For this review, take the finished solid that the model builds, in its own axes (mm). Face numbers are marked on the shaded views. A direction names the side the tool comes from. Round coordinates to 2 decimals unless told otherwise and drop trailing zeros. Order: outer loops, then holes, each group sorted by start corner. A loop starts at its lowest first (then second) coordinate and runs counter-clockwise, first axis right, second up. Notation, with made-up numbers: M 56,-3.5 L 115,-3.5 A21 ccw 115,0.5 Z; hole C -16,42 d5. An arc over 180 degrees is marked long. Use a Markdown table: item, result.
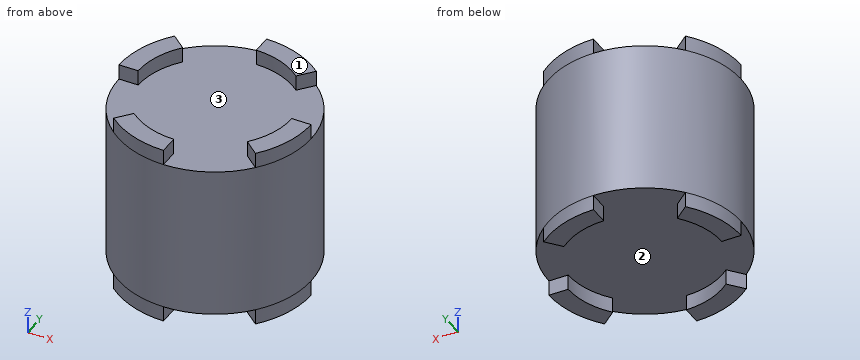
from build123d import *

# Parameters (mm, degrees)
SKETCH1_R           = 25
BOSS_EXTRUDE1_DEPTH = 20
BOSS_EXTRUDE2_START = 4
BOSS_EXTRUDE2_DEPTH = 4


with BuildPart() as part:
    # Sketch1 → Boss-Extrude1 (new, symmetric)
    with BuildSketch(Plane.XY):
        Circle(SKETCH1_R)
    extrude(amount=BOSS_EXTRUDE1_DEPTH, both=True)

    # Sketch2 → Boss-Extrude2 (add)
    with BuildSketch(Plane.XY.offset(20).offset(BOSS_EXTRUDE2_START)):
        with BuildLine():
            Line((-25, 0), (-20, 0))
            ThreePointArc((-20, 0), (-18.793852416, 6.840402867), (-15.320888862, 12.855752194))
            Line((-15.320888862, 12.855752194), (-19.151111078, 16.069690242))
            ThreePointArc((-19.151111078, 16.069690242), (-23.49231552, 8.550503583), (-25, 0))
        make_face()
        with BuildLine():
            Line((16.069690242, 19.151111078), (12.855752194, 15.320888862))
            ThreePointArc((12.855752194, 15.320888862), (6.840402867, 18.793852416), (0, 20))
            Line((0, 20), (0, 25))
            ThreePointArc((0, 25), (8.550503583, 23.49231552), (16.069690242, 19.151111078))
        make_face()
        with BuildLine():
            Line((25, 0), (20, 0))
            ThreePointArc((20, 0), (18.793852416, -6.840402867), (15.320888862, -12.855752194))
            Line((15.320888862, -12.855752194), (19.151111078, -16.069690242))
            ThreePointArc((19.151111078, -16.069690242), (23.49231552, -8.550503583), (25, 0))
        make_face()
        with BuildLine():
            Line((0, -20), (0, -25))
            ThreePointArc((0, -25), (-8.550503583, -23.49231552), (-16.069690242, -19.151111078))
            Line((-16.069690242, -19.151111078), (-12.855752194, -15.320888862))
            ThreePointArc((-12.855752194, -15.320888862), (-6.840402867, -18.793852416), (0, -20))
        make_face()
    boss_extrude2 = extrude(amount=-BOSS_EXTRUDE2_DEPTH)

    # Mirror1: Boss-Extrude2 across plane
    add(boss_extrude2.mirror(Plane.XY))


solid = part.part
Q1. Machinability: for the marked faces 1, 2 and 3, which of the approach directions +Z, -Z, +X, -X, +Y, -Y give a long, thin tool a straight path to every point of the face, cutting with its end or side? Answer none if there is none.
Determined:
| item | result |
|---|---|
| face 1 | +Z, +X, -X, +Y, -Y |
| face 2 | -Z |
| face 3 | +Z |
Q2. Add section A-A (x = -7.5). Write out the cut boundary in (y, z), then the cut area to 3 significant figures.
Determined:
| item | result |
|---|---|
| outline | M -23.85,-24 L -18.54,-24 L -18.54,-20 L 23.85,-20 L 23.85,20 L -18.54,20 L -18.54,24 L -23.85,24 Z |
| area | 1,950 mm^2 |
Q3. Add section B-B (z = -3.5). Write out the cut boundary in (x, y).
Determined:
| item | result |
|---|---|
| outline | C 0,0 d50 |
Q4. Add section C-C (y = 9). Write out the cut boundary in (x, z).
Determined:
| item | result |
|---|---|
| outline | M -23.32,-24 L -17.86,-24 L -17.86,-20 L 23.32,-20 L 23.32,20 L -17.86,20 L -17.86,24 L -23.32,24 Z |
Q5. Clearance check with flat-ended pins moving along their axes: pin 1 (12 mm diameter, centred on x = -19.5, z = -14.5, fed in from -Y); pin 2 (4.5 mm diameter, centred on y = -23.5, z = -22.5, fed in from +X); pin 3 (1 mm diameter, centred on x = -4, y = -8, fed in from +Z); pin 4 (25 mm diameter, centred on x = -12, y = -1.5, fed in from +Z). State where each tip first meets the part, or that it passes through.
Determined:
| item | result |
|---|---|
| pin 1 | stops at y = -21.04 |
| pin 2 | stops at x = 0 |
| pin 3 | stops at z = 20 |
| pin 4 | stops at z = 24 |
Q6. Wall thickness on line 1 along Z through (x, y) = (-17, 15.5); line 2 along X through (y, z) = (8, 8.5); line 3 along Y through (x, z) = (-7.5, -16.5): over which ranges is each line inside the solid? List them lowest first. Write a range as [from, to].
Determined:
| item | result |
|---|---|
| line 1 | z = [-20, 20] |
| line 2 | x = [-23.69, 23.69] |
| line 3 | y = [-23.85, 23.85] |
Q7. Add section D-D (x = -18). Write out the cut boundary in (y, z).
Determined:
| item | result |
|---|---|
| outline | M -17.35,-20 L 8.72,-20 L 8.72,-24 L 15.1,-24 L 15.1,-20 L 17.35,-20 L 17.35,20 L 15.1,20 L 15.1,24 L 8.72,24 L 8.72,20 L -17.35,20 Z |
